Verification items for the finished model (mm, model axes). Give positions to 0.01 mm unless a question says otherwise; leave off trailing zeros. Order: outer loops, then holes, each group sorted by start corner. A loop starts at its lowest first (then second) coordinate and runs counter-clockwise, first axis right, second up. Notation, with made-up numbers: (11, 17.5) -> (31, 17.5) arc R29 ccw to (31, 53.5) -> close; hole circle Ø6 at (34.25, -5.75). An arc over 180 degrees is marked (long way). Write each question's results on one line, items separated by ' | '. Start each with the question number.
1. Mould release check, pull along Y, two halves, no side actions. Record for faces 1 (the face through (76.61, 41.38, 2.17)), 2 (the face through (53.506, 43.133, 2.169)), 3 (the face through (78.771, 10.334, 2.169)), 4 (the face through (9.862, 25.033, 2.169)): +Y half, -Y half, draft (parallel to the pull), parting line (faces both ways), or undercut.
2. Cross-section at A-A, the plane x = 9. Enter the section's corners in (y, z) (3 decimals), then the cut area to 3 significant figures.
3. Cross-section at C-C, the plane z = 1.9. Enter the section's corners in (x, y), then the cut area to 3 significant figures.
4. Depth check by flat-ended pin: pin 1 Ø1 at (x, z) = (38, 1.5) entering from -Y; pin 2 Ø1.5 at (x, z) = (35.5, 1.5) entering from +Y; pin 3 Ø10 at (x, y) = (38, 12) entering from -Z. Enter the tip coordinate at first touch or a pass-through.
5. Cross-section at D-D, the plane x = 52. Enter the section's corners in (y, z), then the cut area to 3 significant figures.
6. Material ranges on L1, parallel to X at y = 29.5, z = 1.55; L2, parallel to X at y = 15, z = 3.15; L3, parallel to Y at x = 101, z = 1.3, recorded low to high. Write a range as from..to.
7. Cross-section at B-B, the plane y = 44. Enter the section's corners in (x, z).
Autodesk Inventor part; units mm, degrees
ref_plane "YZ Plane" through (0, 0, 0) normal (1, 0, 0) x (0, 1, 0)
ref_plane "XZ Plane" through (0, 0, 0) normal (0, 1, 0) x (-1, 0, 0)
ref_plane "XY Plane" through (0, 0, 0) normal (0, 0, 1) x (1, 0, 0)
ref_plane "Work Plane1" through (0, 0, 0) normal (0, 0, 1) x (1, 0, 0)
sketch "Sketch1" plane through (0, 0, 0) normal (0, 0, 1) x (1, 0, 0)
  circle A0 centre (91.7273, 29.791) radius 19.05
  circle A1 centre (39.6359, 28.4758) radius 3
  arc A2 (69.9962, 12.7276) -> (6.7276, 11.146) centre (39.6359, -39.0242) ccw
  arc A3 (69.9962, 12.7276) -> (71.0345, 12.3011) centre (72.0202, 16.1778) ccw
  line L0 (86.2932, 8.4211) -> (71.0345, 12.3011)
  arc A4 (86.2932, 8.4211) -> (86.4826, 51.2082) centre (91.7273, 29.791) ccw
  line L1 (21.44, 35.2803) -> (86.4826, 51.2082)
  arc A5 (21.44, 35.2803) -> (-3.5721, 24.1052) centre (39.6359, -39.0242) ccw
  line L2 (6.7276, 11.146) -> (-3.5721, 24.1052)
  circle A6 centre (10.4041, 22.5922) radius 2.5
  point P0 (0, 0)
extrude "Extrusion1" add sketch "Sketch1" along normal blind 4.4
properties part number "FrontMotorPlateB"
Results below:
1) face 1: undercut | face 2: +Y half | face 3: -Y half | face 4: undercut
2) outline: (12.565, 0) -> (20.524, 0) -> (20.524, 4.4) -> (12.565, 4.4) -> close; (24.661, 0) -> (31.074, 0) -> (31.074, 4.4) -> (24.661, 4.4) -> close | area: 63.2 mm²
3) outline: (-3.57, 24.11) -> (6.73, 11.15) arc R60 cw to (70, 12.73) arc R4 ccw to (71.03, 12.3) -> (86.29, 8.42) arc R22.05 ccw (long way) to (86.48, 51.21) -> (21.44, 35.28) arc R76.5 ccw to start; hole circle Ø5 at (10.4, 22.59); hole circle Ø6 at (39.64, 28.48); hole circle Ø38.1 at (91.73, 29.79) | area: 1,890 mm²
4) pin 1: stops at y = 20.94 | pin 2: stops at y = 38.91 | pin 3: passes through
5) outline: (19.69, 0) -> (42.76, 0) -> (42.76, 4.4) -> (19.69, 4.4) -> close | area: 102 mm²
6) L1: x = 5.63..36.82, 42.46..72.68, 110.78..113.78 | L2: x = 3.66..13.53, 65.74..79.72, 103.73..108.08 | L3: y = 9.79..13.15, 46.43..49.8
7) outline: (57.05, 0) -> (79.04, 0) -> (79.04, 4.4) -> (57.05, 4.4) -> close; (104.42, 0) -> (108.59, 0) -> (108.59, 4.4) -> (104.42, 4.4) -> close
